CAD build for the part. Positions are in the model's coordinates, mm. Round coordinates to 2 decimals unless told otherwise and drop trailing zeros. Order: outer loops, then holes, each group sorted by start corner. A loop starts at its lowest first (then second) coordinate and runs counter-clockwise, first axis right, second up. Notation, with made-up numbers: M 78,79.25 L 134,79.25 A20 ccw 134,100.25 Z; hole C 77,63.5 d11. An arc over 180 degrees is marked long. Put each result on its own line as item: value.
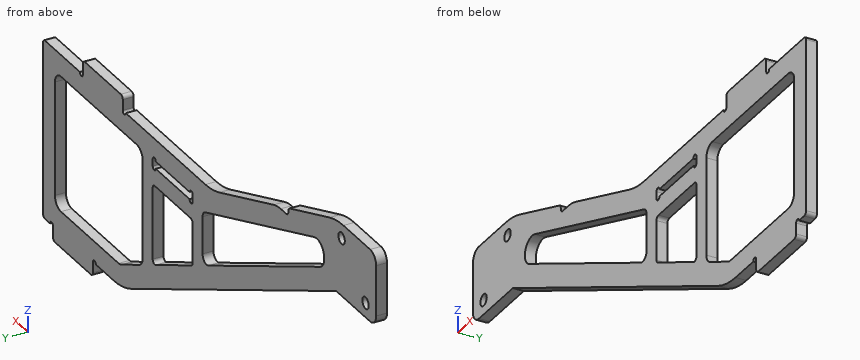
```python
from build123d import *

# Parameters (mm, degrees)
SKETCH_1_R          = 1.6
SKETCH_1_W          = 20
SKETCH_1_H          = 2
EXTRUDE_1_DEPTH     = 3
SKETCH_2_R          = 0.75
CUT_EXTRUDE_1_DEPTH = 157.461656645
FILLET_1_R          = 3
FILLET_2_R          = 20
FILLET_3_R          = 1
FILLET_4_R          = 10


with BuildPart() as part:
    # 草图1 → 凸台-拉伸1 (new body)
    with BuildSketch(Plane(origin=(0, 0, 0), x_dir=(1, 0, 0), z_dir=(0, 1, 0))):
        Polygon((0, 0), (20, 0), (20, 49.5), (15, 49.5), (15, 53.5), (-5, 53.5), (-5, 49.5), (-20, 49.5), (-127, -3), (-147, -3), (-147, -23), (-127, -23), (-103, -14.096774194), (-103, -12), (-97.347826087, -12), (-65, 0), (-20, 0), (-20, -4), (0, -4), align=None)
        with Locations(Location((-141.7, -7, 0), (0, 0, 270))):
            Circle(SKETCH_1_R, mode=Mode.SUBTRACT)
        with Locations(Location((-129.7, -19, 0), (0, 0, 270))):
            Circle(SKETCH_1_R, mode=Mode.SUBTRACT)
        with Locations((-45, 7)):
            Rectangle(SKETCH_1_W, SKETCH_1_H, mode=Mode.SUBTRACT)
    extrude(amount=EXTRUDE_1_DEPTH)

    # 草图2 → 切除-拉伸1 (cut, through all)
    with BuildSketch(Plane(origin=(0, 3, 0), x_dir=(1, 0, 0), z_dir=(0, 1, 0))):
        with Locations((-5.75, 49.5)):
            Circle(SKETCH_2_R)
        with Locations((15.75, 49.5)):
            Circle(SKETCH_2_R)
        with Locations((0.75, 0)):
            Circle(SKETCH_2_R)
        with Locations((-20.75, 0)):
            Circle(SKETCH_2_R)
        with Locations((-54.25, 8)):
            Circle(SKETCH_2_R)
        with Locations((-54.25, 6)):
            Circle(SKETCH_2_R)
        with Locations((-35.75, 6)):
            Circle(SKETCH_2_R)
        with Locations((-35.75, 8)):
            Circle(SKETCH_2_R)
        Polygon((14, 6), (-30, 6), (-30, 37.910143214), (-18.607339503, 43.5), (14, 43.5), align=None)
        Polygon((-35, 35.456872186), (-35, 13), (-55, 13), (-55, 25.643788074), align=None)
        with BuildLine():
            Line((-60, 9.645633867), (-60, 19.981437058))
            ThreePointArc((-60, 19.981437058), (-60.942161442, 21.678781332), (-62.880977584, 21.776953278))
            Line((-62.880977584, 21.776953278), (-118.927003728, -5.722265157))
            ThreePointArc((-118.927003728, -5.722265157), (-120.699269674, -10.510654148), (-116.006358262, -12.522165568))
            Line((-116.006358262, -12.522165568), (-61.304386354, 7.77050143))
            ThreePointArc((-61.304386354, 7.77050143), (-60.358167595, 8.503536518), (-60, 9.645633867))
        make_face()
    extrude(amount=-CUT_EXTRUDE_1_DEPTH, mode=Mode.SUBTRACT)

    # 圆角1
    fillet_1_edges = [part.edges().sort_by_distance(p)[0] for p in [
        (14, 1.5, -43.5),
        (14, 1.5, -6),
        (-30, 1.5, -6),
        (-30, 1.5, -37.910143214),
        (-18.607339503, 1.5, -43.5),
        (-147, 1.5, 23),
        (-147, 1.5, 3),
    ]]
    fillet(fillet_1_edges, radius=FILLET_1_R)

    # 圆角2
    fillet_2_edges = [part.edges().sort_by_distance(p)[0] for p in [
        (-65, 1.5, 0),
        (-127, 1.5, 23),
        (-20, 1.5, -49.5),
    ]]
    fillet(fillet_2_edges, radius=FILLET_2_R)

    # 圆角3
    fillet_3_edges = [part.edges().sort_by_distance(p)[0] for p in [
        (-55, 1.5, -13),
        (-55, 1.5, -25.643788074),
        (-35, 1.5, -35.456872186),
        (-35, 1.5, -13),
        (0, 1.5, 4),
        (-20, 1.5, 4),
        (-103, 1.5, 12),
        (-103, 1.5, 14.096774194),
        (-5, 1.5, -53.5),
        (15, 1.5, -53.5),
        (20, 1.5, -49.5),
        (20, 1.5, 0),
    ]]
    fillet(fillet_3_edges, radius=FILLET_3_R)

    # 圆角4
    fillet_4_edges = [part.edges().sort_by_distance(p)[0] for p in [
        (-97.347826087, 1.5, 12),
    ]]
    fillet(fillet_4_edges, radius=FILLET_4_R)


solid = part.part
```
Item 1: Band-saw the part on A-A on x = -141.7. Give the cut face in (y, z).
Answers below:
outline: M 0,3 L 3,3 L 3,5.4 L 0,5.4 Z; M 0,8.6 L 3,8.6 L 3,23 L 0,23 Z
Item 2: Band-saw the part on D-D on x = -11. Give the cut face in (y, z).
Answers below:
outline: M 0,-49.5 L 3,-49.5 L 3,-43.5 L 0,-43.5 Z; M 0,-6 L 3,-6 L 3,4 L 0,4 Z
Item 3: Band-saw the part on B-B on y = 1.7. State how many separate pieces and enclosed holes the cut face has, and give its area (3 significant figures).
Answers below:
separate pieces: 1
enclosed holes: 6
area: 3,020 mm²
Item 4: Band-saw the part on C-C on x = -45. Give the cut face in (y, z), and give its area (4 significant figures).
Answers below:
outline: M 0,-37.23 L 3,-37.23 L 3,-30.55 L 0,-30.55 Z; M 0,-13 L 3,-13 L 3,-8 L 0,-8 Z; M 0,-6 L 3,-6 L 3,0 L 0,0 Z
area: 53.05 mm²
Item 5: Pin check, flat tips, straight feed: P1, Ø0.6, axis at y = 1, z = -7, coming from the -X side; P2, Ø1.5, axis at x = -28.5, y = 2.5, coming from the -Z side; P3, Ø1.5, axis at y = 1, z = -18, coming from the -X side; P4, Ø4, axis at x = -141.7, z = 7, coming from the -Y side. Stop position of each tip, or through.
Answers below:
P1: x = -107.23
P2: z = -45.7
P3: x = -85.73
P4: y = 0
Item 6: Probe line 1 along Z through (x, y) = (-141.7, 1.5); line 2 along Z through (x, y) = (-129.7, 1.55); line 3 along X through (y, z) = (1.85, -20). List the from-to ranges inside material, lowest first. Write a range as [from, to].
Answers below:
line 1: [3, 5.4], [8.6, 23]
line 2: [3, 17.4], [20.6, 22.98]
line 3: [-80.12, -66.5], [-60, -55], [-35, -30], [14, 20]
